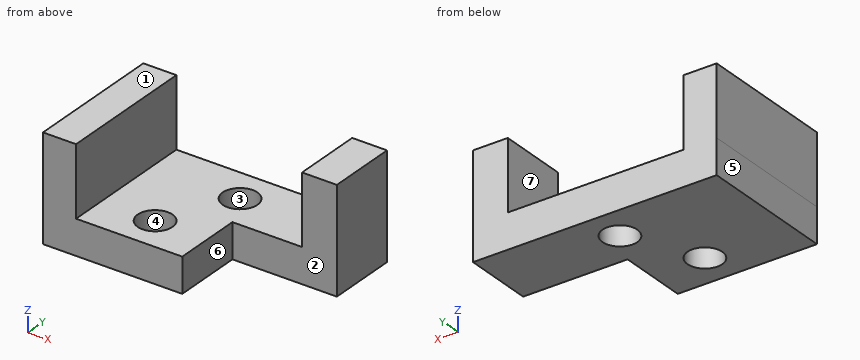
```python
from build123d import *

# Parameters (mm, degrees)
F1_DEPTH = 10
F2_W     = 9.492815
F2_H     = 40
F3_DEPTH = 20
F4_W     = 10
F4_H     = 20
F5_DEPTH = 20
F6_R     = 5
F7_DEPTH = 10.001
F8_R     = 5
F9_DEPTH = 10.001


with BuildPart() as f1:
    # F0 (on Top) → F1 (new body)
    with BuildSketch(Plane.XY):
        Polygon((0, 40), (0, 0), (40, 0), (40, 20), (70, 20), (70, 40), align=None)
    extrude(amount=F1_DEPTH)

    # F2 (on face) → F3 (join)
    with BuildSketch(Plane.XY.offset(10)):
        with Locations((4.746408, 20)):
            Rectangle(F2_W, F2_H)
    extrude(amount=F3_DEPTH)

    # F4 (on face) → F5 (join)
    with BuildSketch(Plane.XY.offset(10)):
        with Locations((65, 30)):
            Rectangle(F4_W, F4_H)
    extrude(amount=F5_DEPTH)

    # F6 (on face) → F7 (cut, through all)
    with BuildSketch(Plane.XY.offset(10)):
        with Locations((25, 10)):
            Circle(F6_R)
    extrude(amount=-F7_DEPTH, mode=Mode.SUBTRACT)

    # F8 (on face) → F9 (cut, through all)
    with BuildSketch(Plane.XY.offset(10)):
        with Locations((35, 30)):
            Circle(F8_R)
    extrude(amount=-F9_DEPTH, mode=Mode.SUBTRACT)


solid = f1.part
```
CAD build for the part. Positions are in the model's coordinates, mm. Face numbers are marked on the shaded views. A direction names the side the tool comes from. Coordinates: 2 decimals unless noted, no trailing zeros. Write each loop counter-clockwise with the first axis right and the second up, starting at its lowest first coordinate (ties: lowest second). Pieces come first, ordered by that corner, then holes. Notation, with made-up numbers: (70, 86.25) -> (118, 86.25) arc R9 ccw to (118, 103.25) -> close; hole circle Ø4 at (-20.5, 69.25). An arc over 180 degrees is marked (long way). Use CSV: the item, a comma, the result in double quotes. Start each with the question number.
Item 1: Tool access for the marked faces 5, 6 and 7: list every direction of +Z, -Z, +X, -X, +Y, -Y with a clear straight run to the whole face (end or side of a thin tool).
Item 2: Band-saw the part on C-C, the plane x = 25. Write the cut outline in (y, z), plus the area to 3 significant figures.
Item 3: Band-saw the part on A-A, the plane z = 22.25. Write the cut outline in (x, y).
Item 4: Band-saw the part on D-D, the plane z = 8.5. Write the cut outline in (x, y), plus the area to 3 significant figures.
Item 5: Two-plate mould, pull along Y, no slides. Class the marked faces 1, 2, 3 and 4: +Y half, -Y half, draft (parallel to the pull), parting line (faces both ways), or undercut.
Item 6: Wall check: probe 1 along Y at (x, z) = (25, 3.75); probe 2 along Y at (x, z) = (35, 2.75); probe 3 along Z at (x, y) = (35.5, 4). Give the ranges that are in metal, low to high.
Item 7: Band-saw the part on B-B, the plane y = 27. Write the cut outline in (x, z), plus the area to 3 significant figures.
Item 8: Drop flat-ended pins along their axis: P1, Ø12, axis at y = 7.5, z = 6, coming from the +X side; P2, Ø8, axis at y = 27.5, z = 3.5, coming from the -X side; P3, Ø20, axis at x = 37, y = 15, coming from the +Z side; P4, Ø15, axis at x = 58, z = 8.5, coming from the -Y side. Give the stop position or say it passes through.
Response values:
1,face 5,"+Z, -Z, -X, +Y, -Y"
1,face 6,"+Z, -Z, +X, -Y"
1,face 7,"+Z, +Y, -Y"
2,outline,"(0, 0) -> (5, 0) -> (5, 10) -> (0, 10) -> close; (15, 0) -> (40, 0) -> (40, 10) -> (15, 10) -> close"
2,area,"300 mm2"
3,outline,"(0, 0) -> (9.49, 0) -> (9.49, 40) -> (0, 40) -> close; (60, 20) -> (70, 20) -> (70, 40) -> (60, 40) -> close"
4,outline,"(0, 0) -> (40, 0) -> (40, 20) -> (70, 20) -> (70, 40) -> (0, 40) -> close; hole circle Ø10 at (25, 10); hole circle Ø10 at (35, 30)"
4,area,"2,040 mm2"
5,face 1,"draft"
5,face 2,"-Y half"
5,face 3,"undercut"
5,face 4,"undercut"
6,probe 1,"y = 0 to 5, 15 to 40"
6,probe 2,"y = 0 to 25, 35 to 40"
6,probe 3,"z = 0 to 10"
7,outline,"(0, 0) -> (31, 0) -> (31, 10) -> (9.49, 10) -> (9.49, 30) -> (0, 30) -> close; (39, 0) -> (70, 0) -> (70, 30) -> (60, 30) -> (60, 10) -> (39, 10) -> close"
7,area,"1,010 mm2"
8,P1,"stops at x = 40"
8,P2,"stops at x = 0"
8,P3,"stops at z = 10"
8,P4,"stops at y = 20"
